Check sheet for the modelled part. Datum: model origin and axes. Units: mm. A direction names the side the tool comes from. Round coordinates to 2 decimals unless told otherwise and drop trailing zeros. Write each loop counter-clockwise with the first axis right and the second up, starting at its lowest first coordinate (ties: lowest second). Pieces come first, ordered by that corner, then holes. Notation, with made-up numbers: (9, 77) - (28, 77) arc R24 ccw to (28, 91) - close; hole circle Ø2 at (-6, -24). An arc over 180 degrees is marked (long way). Use one line per item in the form item = value. Start each with the question number.
1) Gauge pin test, flat ends, axial feed: P1, Ø12, axis at x = 15.5, z = -98, coming from the +Y side; P2, Ø14, axis at y = -83.5, z = -310, coming from the +X side; P3, Ø0.6, axis at x = 1.5, y = -156.5, coming from the +Z side; P4, Ø6, axis at y = -176.5, z = -64.5, coming from the +X side. Record the tip position at first contact, or that the pin passes through.
2) Set-up check for faces 4 (the face through (27, -99, -109)), 5 (the face through (33, -99, -13)), 6 (the face through (8, -99, -233)), 7 (the face through (27, -99, -320)): record each of +Z, -Z, +X, -X, +Y, -Y from which the full face is reachable in a straight line by a thin tool's end or side.
3) Section check C-C (z = -320). Record the boundary of the cut face in (x, y), then the cut area to 3 significant figures.
4) Draft check along Z on faces 1 (the face through (13, -99, -345)), 2 (the face through (10, -200, -184)), 3 (the face through (2, -99, -175)). Enter one of: +Z half, -Z half, draft (parallel to the pull), parting line (faces both ways), or undercut.
5) Section check D-D (z = -26.5). Record the boundary of the cut face in (x, y), then the cut area to 3 significant figures.
6) Section check B-B (x = 18.5). Record the boundary of the cut face in (y, z), then the cut area to 3 significant figures.
7) Scan lines: probe 1 along X at (y, z) = (-76, -201); probe 2 along X at (y, z) = (-88, -17); probe 3 along Z at (x, y) = (3.5, -145.5). Record each from-to range of solid material in increasing order.
8) Section check A-A (z = -63). Record the boundary of the cut face in (x, y), then the cut area to 3 significant figures.
from build123d import *

# Parameters (mm, degrees)
F1_DEPTH = 200
F2_R     = 2
F4_DEPTH = 4
F6_D     = 5
F6_DEPTH = 2


with BuildPart() as f1:
    # F0 (on Front) → F1 (new body)
    with BuildSketch(Plane.XZ):
        Polygon((35, 0), (0, 0), (0, -345), (27, -345), (27, -295), (8, -272.356682), (8, -192.356682), (29, -134.659656), (29, -84.659656), (27, -84.659656), (27, -134.307002), (6, -192.004028), (6, -273.084622), (25, -295.72794), (25, -343), (2, -343), (2, -2), (33, -2), (33, -23), (35, -23), align=None)
    extrude(amount=F1_DEPTH)

    # F2
    f2_edges = [f1.edges().sort_by_distance(p)[0] for p in [
        (0, -100, 0),
        (35, -100, 0),
        (33, -100, -2),
        (2, -100, -2),
        (0, -100, -345),
        (2, -100, -343),
        (27, -100, -345),
        (25, -100, -343),
        (25, -100, -295.72794),
        (27, -100, -295),
        (8, -100, -272.356682),
        (6, -100, -273.084622),
        (6, -100, -192.004028),
        (8, -100, -192.356682),
        (29, -100, -134.659656),
        (27, -100, -134.307002),
    ]]
    fillet(f2_edges, radius=F2_R)

    # F3 (on face) → F4 (cut)
    with BuildSketch(Plane(origin=(0, 0, 0), x_dir=(0, -1, 0), z_dir=(-1, 0, 0))):
        with BuildLine():
            Line((70, -50), (30, -50))
            ThreePointArc((30, -50), (26.464466, -51.464466), (25, -55))
            Line((25, -55), (25, -290))
            ThreePointArc((25, -290), (26.464466, -293.535534), (30, -295))
            Line((30, -295), (70, -295))
            ThreePointArc((70, -295), (73.535534, -293.535534), (75, -290))
            Line((75, -290), (75, -55))
            ThreePointArc((75, -55), (73.535534, -51.464466), (70, -50))
        make_face()
        with BuildLine():
            ThreePointArc((130, -50), (126.464466, -51.464466), (125, -55))
            Line((125, -55), (125, -290))
            ThreePointArc((125, -290), (126.464466, -293.535534), (130, -295))
            Line((130, -295), (170, -295))
            ThreePointArc((170, -295), (173.535534, -293.535534), (175, -290))
            Line((175, -290), (175, -55))
            ThreePointArc((175, -55), (173.535534, -51.464466), (170, -50))
            Line((170, -50), (130, -50))
        make_face()
    extrude(amount=-F4_DEPTH, mode=Mode.SUBTRACT)

    # F6
    with Locations(Plane(origin=(27, 0, 0), x_dir=(0, -1, 0), z_dir=(-1, 0, 0))):
        with Locations((50, -109.307002), (150, -109.307002)):
            Hole(F6_D / 2, depth=F6_DEPTH)


solid = f1.part
Results are:
q1.P1 = through
q1.P2 = 27
q1.P3 = -0.01
q1.P4 = 2
q2.face_4 = +Y, -Y
q2.face_5 = -Z, +Y, -Y
q2.face_6 = +X, +Y, -Y
q2.face_7 = -Z, +X, +Y, -Y
q3.outline = (0, -200) - (2, -200) - (2, 0) - (0, 0) - close; (25, -200) - (27, -200) - (27, 0) - (25, 0) - close
q3.area = 800 mm²
q4.face_1 = -Z half
q4.face_2 = draft
q4.face_3 = undercut
q5.outline = (0, -200) - (2, -200) - (2, 0) - (0, 0) - close
q5.area = 400 mm²
q6.outline = (-200, -345) - (0, -345) - (0, -343) - (-200, -343) - close; (-200, -287.98) - (0, -287.98) - (0, -284.87) - (-200, -284.87) - close; (-200, -163.51) - (0, -163.51) - (0, -157.66) - (-200, -157.66) - close; (-200, -2) - (0, -2) - (0, 0) - (-200, 0) - close
q6.area = 2,590 mm²
q7.probe_1 = 0 to 2, 6 to 8
q7.probe_2 = 0 to 2, 33 to 35
q7.probe_3 = -345 to -342.94, -2.06 to 0
q8.outline = (0, -200) - (2, -200) - (2, -175) - (0, -175) - close; (0, -125) - (2, -125) - (2, -75) - (0, -75) - close; (0, -25) - (2, -25) - (2, 0) - (0, 0) - close
q8.area = 200 mm²
